Job drawing, mm, ordinate dimensions from the low corner. One solid piece. Round coordinates to 2 decimals unless told otherwise and drop trailing zeros. Order: outer loops, then holes, each group sorted by start corner. A loop starts at its lowest first (then second) coordinate and runs counter-clockwise, first axis right, second up. Notation, with made-up numbers: (25.5, 4) -> (57.5, 4) arc R35 cw to (57.5, 43) -> close; hole circle Ø5 at (-25, 44.25). An arc over 180 degrees is marked (long way). Write item = value, one per line.
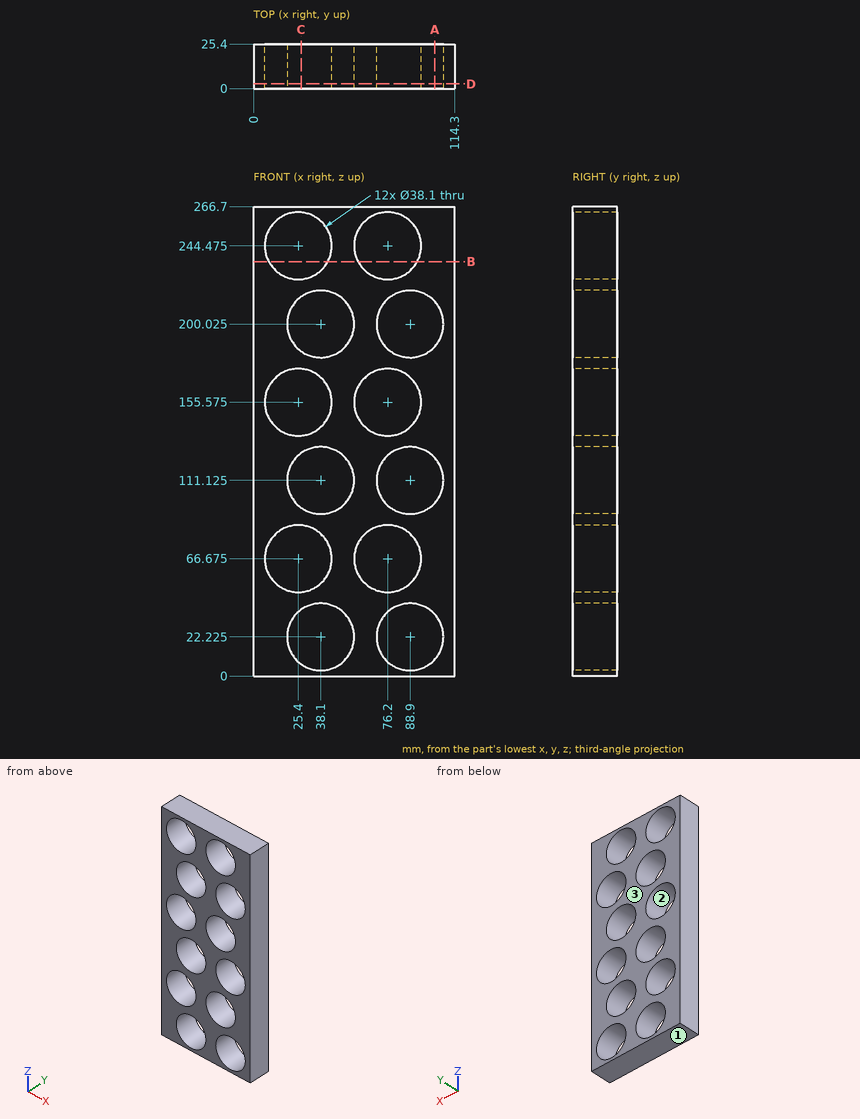
Q1. Cut at A-A, the plane x = 103. List the corners of the cut face in (y, z).
Check values:
outline = (0, 0) -> (25.4, 0) -> (25.4, 9.42) -> (0, 9.42) -> close; (0, 35.03) -> (25.4, 35.03) -> (25.4, 98.32) -> (0, 98.32) -> close; (0, 123.93) -> (25.4, 123.93) -> (25.4, 187.22) -> (0, 187.22) -> close; (0, 212.83) -> (25.4, 212.83) -> (25.4, 266.7) -> (0, 266.7) -> close
Q2. Cut at B-B, the plane z = 235.5. List the corners of the cut face in (x, y).
Check values:
outline = (0, 0) -> (8.6, 0) -> (8.6, 25.4) -> (0, 25.4) -> close; (42.2, 0) -> (59.4, 0) -> (59.4, 25.4) -> (42.2, 25.4) -> close; (93, 0) -> (114.3, 0) -> (114.3, 25.4) -> (93, 25.4) -> close
Q3. Cut at C-C, the plane x = 27. List the corners of the cut face in (y, z).
Check values:
outline = (0, 0) -> (25.4, 0) -> (25.4, 6.74) -> (0, 6.74) -> close; (0, 37.71) -> (25.4, 37.71) -> (25.4, 47.69) -> (0, 47.69) -> close; (0, 85.66) -> (25.4, 85.66) -> (25.4, 95.64) -> (0, 95.64) -> close; (0, 126.61) -> (25.4, 126.61) -> (25.4, 136.59) -> (0, 136.59) -> close; (0, 174.56) -> (25.4, 174.56) -> (25.4, 184.54) -> (0, 184.54) -> close; (0, 215.51) -> (25.4, 215.51) -> (25.4, 225.49) -> (0, 225.49) -> close; (0, 263.46) -> (25.4, 263.46) -> (25.4, 266.7) -> (0, 266.7) -> close
Q4. Flat gauge pin, fed straight in: pin 1 (8 mm diameter, centred on x = 69.5, z = 232, fed in from -Y). Where does the tip first touch, or does it go through?
Check values:
pin_1 = through
Q5. Probe probe 1 along X at (y, z) = (14.25, 111); probe 2 along X at (y, z) = (2.75, 157); probe 3 along Z at (x, y) = (68, 6.75). List the from-to ranges inside material, lowest first.
Check values:
probe_1 = 0 to 19.05, 57.15 to 69.85, 107.95 to 114.3
probe_2 = 0 to 6.4, 44.4 to 57.2, 95.2 to 114.3
probe_3 = 0 to 49.48, 83.87 to 138.38, 172.77 to 227.28, 261.67 to 266.7
Q6. Cut at D-D, the plane y = 2.75. Give the number of separate pieces and of enclosed holes in the cut face, and give its area (3 significant figures).
Check values:
separate_pieces = 1
enclosed_holes = 12
area = 16,800 mm²
Q7. Mould opens along Z. For the marked faces 1, 2 and 3 say: released by +Z, released by -Z, zero draft, split by the parting line, or undercut.
Check values:
face_1 = released by -Z
face_2 = undercut
face_3 = zero draft
